Here's how the part is built. I have some questions about the finished solid (model axes, mm). A direction names the side the tool comes from. Coordinates: 2 decimals unless noted, no trailing zeros. Loops run counter-clockwise (first coordinate to the right, second up) from the corner with the lowest first, then second, coordinate; pieces in that order, holes last. Notation, with made-up numbers: (13.5, -35.75) -> (50.5, -35.75) arc R14 ccw to (50.5, -11.75) -> close; hole circle Ø3 at (57, 89). An arc over 180 degrees is marked (long way). Answer as a JSON object with one key per item and string values. Group by question number.
Q1. On a 3-axis mill with a long thin cutter (end or side, diameter ignored), from which of +Z, -Z, +X, -X, +Y, -Y can I reach the whole of each face in a straight line? I mean faces 1 (the flat face through (170, 0, 51)), 2 (the flat face through (-170, 0, 51)), 3 (the flat face through (169, 0, 48)). Say none if no direction works.
Q2. I want a section at D-D on x = -110.5. Write out the boundary of the cut face in (y, z), then the cut area to 3 significant figures.
Q3. I need wall thicknesses on line 1 (Y direction, x = -195, z = 0.4); line 2 (Y direction, x = 12, z = 52.5); line 3 (Y direction, x = 68.67, z = 94.75). Which ranges of each line are inside material? Lowest first, please.
Q4. I want a section at C-C on z = 14. Write out the boundary of the cut face in (x, y).
Q5. I want a section at B-B on y = -14.5. Count the separate pieces of the cut face and the enclosed holes in it, then the cut area to 3 significant figures.
Q6. I want a section at A-A on x = -1.33. Write out the boundary of the cut face in (y, z).
Q7. I'm going to push flat-ended pins straight in: pin 1 (10 mm diameter, centred on y = -27.5, z = 46.5, fed in from -X); pin 2 (6 mm diameter, centred on x = -125, y = 10.5, fed in from -Z); pin 3 (9.5 mm diameter, centred on x = 195, y = -25, fed in from -Z); pin 4 (20.5 mm diameter, centred on y = -12, z = 28, fed in from +X). Where does each tip first touch, or does it pass through?
Q8. Thinking about a two-plate mould opening in Y: for faces 4 (the flat face through (190, 0, 1)), 5 (the flat face through (-3, -35, 47)), 6 (the flat face through (-169, 0, 48)), which applies, released by +Y, released by -Y, zero draft, split by the parting line, or undercut?
```python
from build123d import *

# Parameters (mm, degrees)
SKETCH_1_W          = 410
SKETCH_1_H          = 70
EXTRUDE_1_DEPTH     = 95
SKETCH_2_W          = 35
SKETCH_2_H          = 94
CUT_EXTRUDE_1_DEPTH = 95
SHELL_1_T           = -1
FILLET_2_R          = 5
SKETCH_3_R          = 2.9999999999999947
SKETCH_3_R_2        = 2.999999999999994
SKETCH_3_R_3        = 3.000000000000047
CUT_EXTRUDE_2_DEPTH = 229.22357459298556
SKETCH_4_R          = 20.000000000000004
SKETCH_4_R_2        = 20
SKETCH_4_R_3        = 19.999999999999986
CUT_EXTRUDE_3_DEPTH = 229.63726730347355


with BuildPart() as part:
    # 草图1 → 凸台-拉伸1 (new body)
    with BuildSketch(Plane.XY):
        Rectangle(SKETCH_1_W, SKETCH_1_H)
    extrude(amount=EXTRUDE_1_DEPTH)

    # 草图2 → 切除-拉伸1 (cut)
    with BuildSketch(Plane(origin=(0, 34.99999999999999, 0), x_dir=(1, 0, 0), z_dir=(0, 1, 0))):
        with Locations((187.49999999999997, -48)):
            Rectangle(SKETCH_2_W, SKETCH_2_H)
        Polygon((-204.99999999999997, -1.0000000000001206), (-204.99999999999991, -95.00000000000011), (-169.99999999999994, -95.00000000000011), (-169.99999999999997, -1.0000000000001001), align=None)
    extrude(amount=-CUT_EXTRUDE_1_DEPTH, mode=Mode.SUBTRACT)

    # 抽壳1
    shell_1_openings = [part.faces().sort_by_distance(p)[0] for p in [
        (0, 0, 0),
    ]]
    offset(amount=SHELL_1_T, openings=shell_1_openings, kind=Kind.INTERSECTION)

    # 圆角2
    fillet_2_edges = [part.edges().sort_by_distance(p)[0] for p in [
        (169.99999999999997, -7.11e-15, 1.0000000000000009),
        (-169.99999999999997, -7.11e-15, 1.0000000000001001),
    ]]
    fillet(fillet_2_edges, radius=FILLET_2_R)

    # 草图3 → 切除-拉伸2 (cut, through all)
    with BuildSketch(Plane.XY.offset(1.000000000000001)):
        with Locations((194.99999999999994, 24.999999999999993)):
            Circle(SKETCH_3_R)
        with Locations(Location((194.99999999999994, -25.000000000000007, 0), (0, 0, 180))):
            Circle(SKETCH_3_R)
        with Locations((194.99999999999994, -6.94e-15)):
            Circle(SKETCH_3_R_2)
        with Locations(Location((-194.9999999999999, -1.5959e-13, 0), (0, 0, 180))):
            Circle(SKETCH_3_R_3)
        with Locations(Location((-194.99999999999994, 24.999999999999837, 0), (0, 0, 180))):
            Circle(SKETCH_3_R)
        with Locations((-194.9999999999999, -25.00000000000016)):
            Circle(SKETCH_3_R)
    extrude(amount=-CUT_EXTRUDE_2_DEPTH, mode=Mode.SUBTRACT)

    # 草图4 → 切除-拉伸3 (cut, through all)
    with BuildSketch(Plane.XY.offset(95)):
        with Locations((-141.32999999999993, -1.8400000000000152)):
            Circle(SKETCH_4_R)
        with Locations((-71.32999999999993, -1.8400000000000152)):
            Circle(SKETCH_4_R)
        with Locations((-1.3299999999999146, -1.8400000000000152)):
            Circle(SKETCH_4_R_2)
        with Locations((68.67000000000009, -1.8400000000000152)):
            Circle(SKETCH_4_R)
        with Locations((138.6700000000001, -1.8400000000000152)):
            Circle(SKETCH_4_R_3)
    extrude(amount=-CUT_EXTRUDE_3_DEPTH, mode=Mode.SUBTRACT)


solid = part.part
```
Result set:
{
 "1": {"face 1": "+Z, +X, +Y, -Y", "face 2": "+Z, -X, +Y, -Y", "face 3": "-Z"},
 "2": {"outline": "(-35, 0) -> (-34, 0) -> (-34, 94) -> (34, 94) -> (34, 0) -> (35, 0) -> (35, 95) -> (-35, 95) -> close", "area": "258 mm²"},
 "3": {"line 1": "y = -35 to -28, -22 to -3, 3 to 22, 28 to 35", "line 2": "y = -35 to -34, 34 to 35", "line 3": "y = -35 to -21.84, 18.16 to 35"},
 "4": {"outline": "(-170, -35) -> (170, -35) -> (170, 35) -> (-170, 35) -> close; hole (-169, -34) -> (169, -34) -> (169, 34) -> (-169, 34) -> close"},
 "5": {"separate pieces": "6", "enclosed holes": "0", "area": "454 mm²"},
 "6": {"outline": "(-35, 0) -> (-34, 0) -> (-34, 94) -> (-21.84, 94) -> (-21.84, 95) -> (-35, 95) -> close; (18.16, 94) -> (34, 94) -> (34, 0) -> (35, 0) -> (35, 95) -> (18.16, 95) -> close"},
 "7": {"pin 1": "stops at x = -170", "pin 2": "stops at z = 94", "pin 3": "stops at z = 0", "pin 4": "stops at x = 170"},
 "8": {"face 4": "zero draft", "face 5": "released by -Y", "face 6": "undercut"}
}
